```python
from build123d import *

# Parameters (mm, degrees)
F0_W           = 45
F0_H           = 25
F1_DEPTH       = 6
F2_R           = 5
F5_DEPTH       = 25
F6_R           = 2.1
F7_DEPTH       = 25
F9_R           = 7.5
F10_DEPTH      = 5
F10_DEPTH_BACK = 25
F11_W          = 49.2877000943
F11_H          = 30.2235903218
F12_DEPTH      = 25
F13_W          = 37.6632460393
F13_H          = 10.6945014559
F14_DEPTH      = 25
F15_R          = 3
F16_DEPTH      = 25
F16_DEPTH_BACK = 25
F18_R          = 3


# Not quite as in the source:
# - a fillet or chamfer that OpenCascade refuses, or shapes differently, is made with other operations: its cross-section is extruded or revolved along the edge and cut away or added


with BuildPart() as f1:
    # F0 (on Top) → F1 (new body)
    with BuildSketch(Plane.XY):
        with Locations((22.5, 12.5)):
            Rectangle(F0_W, F0_H)
    extrude(amount=F1_DEPTH)

    # F2
    f2_edges = [f1.edges().sort_by_distance(p)[0] for p in [
        (45, 25, 3),
        (45, 0, 3),
        (0, 25, 3),
        (0, 0, 3),
    ]]
    fillet(f2_edges, radius=F2_R)

    # F4 (on offset) → F5 (cut)
    with BuildSketch(Plane.XY.offset(3)):
        Polygon((3, 14.6650635095), (3, 10.3349364905), (6.75, 8.1698729811), (10.5, 10.3349364905), (10.5, 14.6650635095), (6.75, 16.8301270189), align=None)
        Polygon((42, 10.3349364905), (42, 14.6650635095), (38.25, 16.8301270189), (34.5, 14.6650635095), (34.5, 10.3349364905), (38.25, 8.1698729811), align=None)
    extrude(amount=F5_DEPTH, mode=Mode.SUBTRACT)

    # F6 (on Top) → F7 (cut)
    with BuildSketch(Plane.XY):
        with Locations((6.75, 12.5)):
            Circle(F6_R)
        with Locations((38.25, 12.5)):
            Circle(F6_R)
    extrude(amount=F7_DEPTH, mode=Mode.SUBTRACT)

    # F9 (on face) → F10 (join, two sides)
    with BuildSketch(Plane(origin=(0, -2.954423259, 2.479055467), x_dir=(1, 0, 0), z_dir=(0, -0.7660444431, 0.6427876097))) as f10_sk:
        with Locations((22.5, 8)):
            Circle(F9_R)
    extrude(amount=F10_DEPTH)
    extrude(f10_sk.sketch, amount=-F10_DEPTH_BACK)

    # F11 (on Top) → F12 (cut)
    with BuildSketch(Plane.XY):
        with Locations((22.6797270589, 13.7661970221)):
            Rectangle(F11_W, F11_H)
    extrude(amount=-F12_DEPTH, mode=Mode.SUBTRACT)

    # F13 (on face) → F14 (cut)
    with BuildSketch(Plane(origin=(0, 25, 0), x_dir=(-1, 0, 0), z_dir=(0, 1, 0))):
        with Locations((-22.6992729586, 2.3689556401)):
            Rectangle(F13_W, F13_H)
    extrude(amount=F14_DEPTH, mode=Mode.SUBTRACT)

    # F15 (on face) → F16 (cut, two sides)
    with BuildSketch(Plane(origin=(0, -2.954423259, 2.479055467), x_dir=(1, 0, 0), z_dir=(0, -0.7660444431, 0.6427876097))) as f16_sk:
        with Locations((22.5, 8)):
            Circle(F15_R)
    extrude(amount=F16_DEPTH, mode=Mode.SUBTRACT)
    extrude(f16_sk.sketch, amount=-F16_DEPTH_BACK, mode=Mode.SUBTRACT)

    # F17: chamfer of 3 x 5 on 1 edges, made by hand

    # F17_s1 → F17_t2 (revolve, cut)
    with BuildSketch(Plane(origin=(0, 5.1423008775, 6.128355545), x_dir=(1, 0, 0), z_dir=(0, 0.6427876097, 0.7660444431))):
        Polygon((28.5, -8.8567256581), (25.5, -3.8567256581), (25.5, -8.8567256581), align=None)
    revolve(axis=Axis((22.5, -1.6423445971, 11.8213490604), (0, 0.7660444431, -0.6427876097)), mode=Mode.SUBTRACT)

    # F18
    f18_edges = [f1.edges().sort_by_distance(p)[0] for p in [
        (19.5, 2.187878, 8.607411),
    ]]
    fillet(f18_edges, radius=F18_R)

    # F19: fillet of radius 3 on 1 edges, made by hand

    # F19_s1 → F19_t2 (revolve, cut)
    with BuildSketch(Plane(origin=(0, 5.1423008775, 6.128355545), x_dir=(1, 0, 0), z_dir=(0, 0.6427876097, 0.7660444431))):
        with BuildLine():
            ThreePointArc((27.6302051352, -7.4070675501), (28.6371938466, -8.4227287465), (30, -8.8567256581))
            Line((30, -8.8567256581), (28.5, -8.8567256581))
            Line((28.5, -8.8567256581), (27.6302051352, -7.4070675501))
        make_face()
    revolve(axis=Axis((22.5, -1.6423445971, 11.8213490604), (0, 0.7660444431, -0.6427876097)), mode=Mode.SUBTRACT)


solid = f1.part
```
The listing builds one solid part. Answer for the finished solid, in the listing's coordinates (mm). A direction names the side the tool comes from. Give positions to 0.01 mm unless a question says otherwise; leave off trailing zeros. Loops run counter-clockwise (first coordinate to the right, second up) from the corner with the lowest first, then second, coordinate; pieces in that order, holes last. Notation, with made-up numbers: (64, -24) - (92, -24) arc R33 cw to (92, 10) - close; hole circle Ø10 at (-5.75, 44.25). An arc over 180 degrees is marked (long way). Return JSON: item names as keys, results as strings. Group by question number.
1. Straight lines are drawn through the part: line 1 (X direction, y = 12.5, z = 1.6); line 2 (Y direction, x = 38.25, z = 1.3); line 3 (X direction, y = 12.5, z = 0.75). For each, find the intervals that lie inside material, in ascending order. Write a range as [from, to].
2. Given pin 1 Ø5.5 at (x, y) = (38.25, 12.5) entering from +Z; pin 2 Ø6.5 at (x, z) = (28, 2.5) entering from -Y; pin 3 Ø1 at (y, z) = (1, 7.5) entering from -X, each flat-ended and moving along its own axis, determine where each tip first touches the part or whether it passes through.
3. Which of the six approach directions +Z, -Z, +X, -X, +Y, -Y give full straight-line access (tool end or side, diameter ignored) to faces 4 (the flat face through (45, 12, 3)), 5 (the flat face through (40.151, 15.732, 4.479))?
4. Determine the mould class of faces 1 (the flat face through (4.849, 9.268, 4.479)), 2 (the flat face through (22.3, 0, 0.3)), 3 (the cylindrical face through (44, 23, 3)) for opening direction Y: pulls with the +Y half, pulls with the -Y half, needs draft (parallel to the pull), parting line crosses it, or undercut.
5. Find section A-A (x = 12). Write down the section's boundary in (y, z).
6. Find section B-B (z = 1.5). State how many separate pieces and enclosed holes the cut face has, then the cut area to 3 significant figures.
Verdict:
{
 "1": {"line 1": "x = [0, 4.65], [8.85, 19.78], [25.22, 36.15], [40.35, 45]", "line 2": "y = [0, 10.4], [14.6, 25]", "line 3": "x = [0, 4.65], [8.85, 19.56], [25.44, 36.15], [40.35, 45]"},
 "2": {"pin 1": "stops at z = 3", "pin 2": "stops at y = -3.91", "pin 3": "stops at x = 15.08"},
 "3": {"face 4": "+Z, -Z, +X, +Y, -Y", "face 5": "+Z"},
 "4": {"face 1": "undercut", "face 2": "pulls with the -Y half", "face 3": "pulls with the +Y half"},
 "5": {"outline": "(0, 0) - (25, 0) - (25, 6) - (0, 6) - close"},
 "6": {"separate pieces": "1", "enclosed holes": "3", "area": "1,040 mm^2"}
}
